The figure shows three views and two pictorial views of one solid part (mm, origin at its lowest corner). Answer the questions. A direction names the side the tool comes from. Round coordinates to 2 decimals unless told otherwise and drop trailing zeros. Write each loop counter-clockwise with the first axis right and the second up, starting at its lowest first coordinate (ties: lowest second). Pieces come first, ordered by that corner, then holes. Notation, with made-up numbers: M 6,-30.5 L 29,-30.5 A11 cw 29,-16.5 Z; hole C -16,61 d10. An arc over 180 degrees is marked long. Answer in a Markdown table with one row per item.
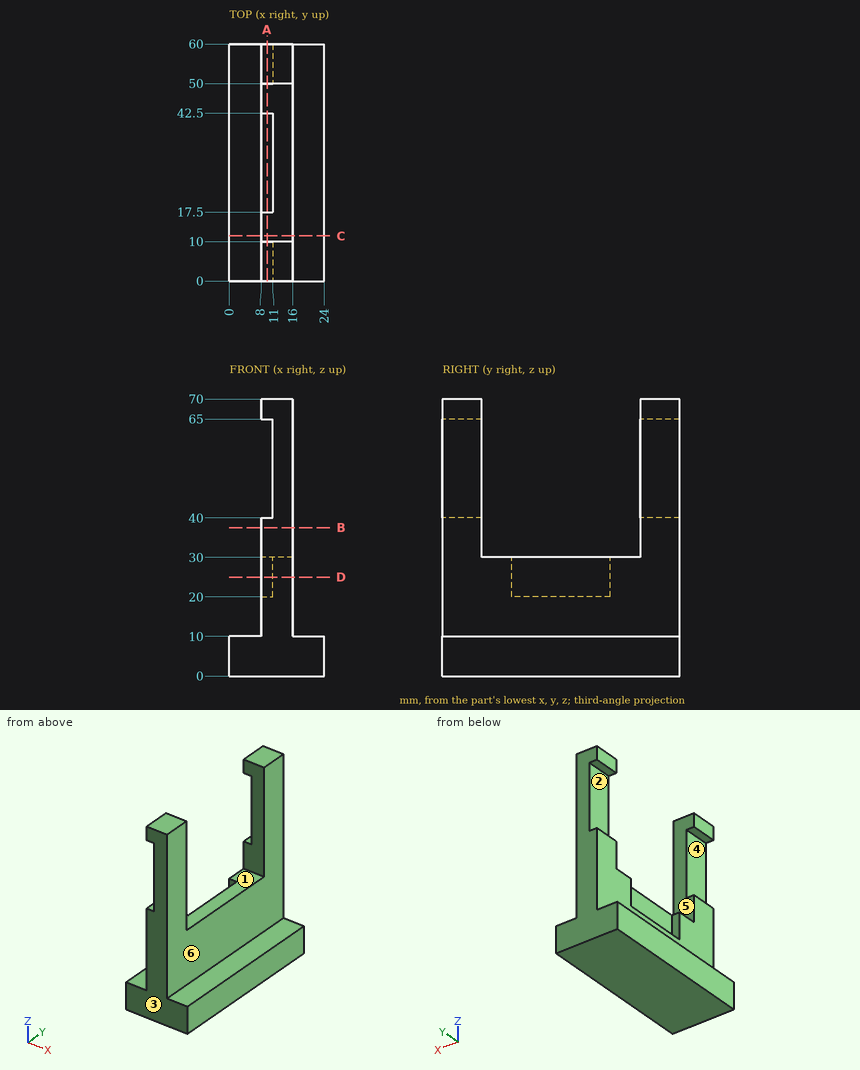
1. Given pin 1 (8 mm diameter, centred on x = 3, z = 21, fed in from -Y); pin 2 (3 mm diameter, centred on y = 53.5, z = 49, fed in from -X); pin 3 (2.5 mm diameter, centred on x = 10, y = 32, fed in from +Z); pin 4 (5.5 mm diameter, centred on y = 56.5, z = 68, fed in from -X), each flat-ended and moving along its own axis, determine where each tip first touches the part or whether it passes through.
Calculated:
| item | result |
|---|---|
| pin 1 | passes through |
| pin 2 | stops at x = 11 |
| pin 3 | stops at z = 30 |
| pin 4 | stops at x = 8 |
2. Consider line 1 along X through (y, z) = (51, 56); line 2 along Z through (x, y) = (2.25, 26.5); line 3 along X through (y, z) = (20, 15). Determine where each line is inside the solid, lowest interval first. Write a range as from..to.
Calculated:
| item | result |
|---|---|
| line 1 | x = 11..16 |
| line 2 | z = 0..10 |
| line 3 | x = 8..16 |
3. The part is cut by section B-B (z = 37.5). Determine the outline of the cut face in (x, y).
Calculated:
| item | result |
|---|---|
| outline | M 8,0 L 16,0 L 16,10 L 8,10 Z; M 8,50 L 16,50 L 16,60 L 8,60 Z |
4. Determine the mould class of the marked faces 1, 2 and 3 for opening direction Y: released by +Y, released by -Y, zero draft, split by the parting line, or undercut.
Calculated:
| item | result |
|---|---|
| face 1 | undercut |
| face 2 | zero draft |
| face 3 | released by -Y |
5. The part is cut by section C-C (y = 11.5). Determine the outline of the cut face in (x, z).
Calculated:
| item | result |
|---|---|
| outline | M 0,0 L 24,0 L 24,10 L 16,10 L 16,30 L 8,30 L 8,10 L 0,10 Z |
6. The part is cut by section A-A (x = 9.5). Determine the outline of the cut face in (y, z), plus the area to 3 significant figures.
Calculated:
| item | result |
|---|---|
| outline | M 0,0 L 60,0 L 60,40 L 50,40 L 50,30 L 42.5,30 L 42.5,20 L 17.5,20 L 17.5,30 L 10,30 L 10,40 L 0,40 Z; M 0,65 L 10,65 L 10,70 L 0,70 Z; M 50,65 L 60,65 L 60,70 L 50,70 Z |
| area | 1,850 mm² |
7. The part is cut by section D-D (z = 25). Determine the outline of the cut face in (x, y), plus the area to 3 significant figures.
Calculated:
| item | result |
|---|---|
| outline | M 8,0 L 16,0 L 16,60 L 8,60 L 8,42.5 L 11,42.5 L 11,17.5 L 8,17.5 Z |
| area | 405 mm² |
8. A tool of negligible diameter and unlimited length cuts with its end or side. For the marked faces 4, 5 and 6, from which of +Z, -Z, +X, -X, +Y, -Y can it reach the whole face along a straight path? Write none if from no direction.
Calculated:
| item | result |
|---|---|
| face 4 | -X, +Y, -Y |
| face 5 | +Z, +X, -X |
| face 6 | +Z, +X, +Y, -Y |
